The model under review builds one solid part; all positions refer to its coordinate system, in mm. A direction names the side the tool comes from. Round coordinates to 2 decimals unless told otherwise and drop trailing zeros. Write each loop counter-clockwise with the first axis right and the second up, starting at its lowest first coordinate (ties: lowest second). Pieces come first, ordered by that corner, then holes. Notation, with made-up numbers: (54, 14.5) -> (88, 14.5) arc R22 ccw to (88, 43.5) -> close; hole circle Ø8 at (16, -22). An arc over 180 degrees is marked (long way). Return JSON: item names as keys, results as strings. Group by question number.
1. Clearance check with flat-ended pins moving along their axes: P1, Ø1.2, axis at x = 47.5, y = -2, coming from the -Z side; P2, Ø0.8, axis at x = 3.5, z = -111.5, coming from the -Y side; P3, Ø0.8, axis at x = 44.5, z = -88, coming from the -Y side; P4, Ø2, axis at x = 47.5, y = -2, coming from the +Z side. State where each tip first meets the part, or that it passes through.
2. Mouldability with a two-part tool opening along Z and no side actions: class faces 4 (the flat face through (47, -2, -85.5)), 5 (the cylindrical face through (62.67, -1.97, -90.48)), 6 (the flat face through (47, -2, -90.5)), 7 (the flat face through (64, -4, -89)) as pulls with the +Z half, pulls with the -Z half, needs draft (parallel to the pull), parting line crosses it, or undercut.
3. Take a section at A-A, the plane y = -2.5. Give the number of separate pieces and of enclosed holes in the cut face, then the cut area to 3 significant figures.
4. Tool access review of faces 1 (the cylindrical face through (52, -2, -22)), 2 (the flat face through (39, 2, 0)), 3 (the flat face through (47, -2, -24.5)): name each direction out of +Z, -Z, +X, -X, +Y, -Y from which nothing blocks a thin tool from reaching the whole face with its end or side.
5. Take a section at B-B, the plane z = -16. Write out the cut boundary in (x, y), then the cut area to 3 significant figures.
6. Take a section at C-C, the plane x = 27. Write out the cut boundary in (y, z).
7. For line 1 along Z through (x, y) = (49.5, -0.9); line 2 along Z through (x, y) = (3.5, 1.9); line 3 along Z through (x, y) = (51.5, -0.5), list the stretches that pass through material, from the lowest coordinate up. Write a range as from..to.
Autodesk Inventor part; units mm, degrees
ref_plane "YZ Plane" through (0, 0, 0) normal (1, 0, 0) x (0, 1, 0)
ref_plane "XZ Plane" through (0, 0, 0) normal (0, 1, 0) x (-1, 0, 0)
ref_plane "XY Plane" through (0, 0, 0) normal (0, 0, 1) x (1, 0, 0)
sketch "Skizze1" plane through (0, 0, 0) normal (0, 1, 0) x (-1, 0, 0)
  line L0 (0, 0) -> (-80, 0)
  line L1 (-80, 0) -> (-80, -115)
  line L2 (-80, -115) -> (0, -115)
  line L3 (0, -115) -> (0, 0)
  line L4 (-3.5, -3.5) -> (-76.5, -3.5) construction
  line L5 (-76.5, -3.5) -> (-76.5, -111.5) construction
  line L6 (-76.5, -111.5) -> (-3.5, -111.5) construction
  line L7 (-3.5, -111.5) -> (-3.5, -3.5) construction
  circle A0 centre (-3.5, -3.5) radius 0.7
  circle A1 centre (-3.5, -111.5) radius 0.7
  circle A2 centre (-76.5, -111.5) radius 0.7
  circle A3 centre (-76.5, -3.5) radius 0.7
  dimension "d0" = 115
  dimension "d1" = 80
  dimension "d2" = 3.5
  dimension "d3" = 1.4
extrude "Extrusion1" add sketch "Skizze1" along normal blind 4
chamfer "Fasen1" distance 1.2 angle 45 4 edges at (4.2, 4, -3.5) (4.2, 4, -111.5) (77.2, 4, -111.5) (77.2, 4, -3.5)
sketch "Skizze2" plane through (0, 0, 0) normal (0, -1, 0) x (1, 0, 0)
  line L0 (29, -90) -> (46.5, -90) construction
  line L1 (46.5, -90) -> (46.5, -20) construction
  line L2 (46.5, -20) -> (29, -20) construction
  line L3 (29, -20) -> (29, -90) construction
  line L4 (0, -115) -> (0, 0) construction
  line L5 (47.5, -90) -> (65, -90) construction
  line L6 (65, -90) -> (65, -20) construction
  line L7 (65, -20) -> (47.5, -20) construction
  line L8 (47.5, -20) -> (47.5, -90) construction
  line L9 (80, -115) -> (0, -115) construction
  circle A0 centre (31, -88) radius 2.5
  arc A1 (44.5, -85.5) -> (44.5, -90.5) centre (44.5, -88) ccw
  circle A2 centre (63, -88) radius 2.5
  circle A3 centre (31, -22) radius 2.5
  arc A4 (44.5, -19.5) -> (44.5, -24.5) centre (44.5, -22) ccw
  arc A5 (49.5, -24.5) -> (49.5, -19.5) centre (49.5, -22) ccw
  circle A6 centre (63, -22) radius 2.5
  line L10 (31, -88) -> (44.5, -88) construction
  line L11 (44.5, -88) -> (44.5, -22) construction
  line L12 (44.5, -22) -> (31, -22) construction
  line L13 (31, -22) -> (31, -88) construction
  line L14 (49.5, -88) -> (63, -88) construction
  line L15 (63, -88) -> (63, -22) construction
  line L16 (63, -22) -> (49.5, -22) construction
  line L17 (49.5, -22) -> (49.5, -88) construction
  line L18 (44.5, -90.5) -> (49.5, -90.5)
  line L19 (44.5, -85.5) -> (49.5, -85.5)
  line L20 (44.5, -24.5) -> (49.5, -24.5)
  line L21 (44.5, -19.5) -> (49.5, -19.5)
  arc A7 (49.5, -90.5) -> (49.5, -85.5) centre (49.5, -88) ccw
  dimension "d9" = 29
  dimension "d10" = 17.5
  dimension "d11" = 70
  dimension "d12" = 25
  dimension "d13" = 1
  dimension "d14" = 2
  dimension "d15" = 2
  dimension "d16" = 5
extrude "Extrusion2" add sketch "Skizze2" along normal blind 4
sketch "Skizze3" plane through (31, -4, -22) normal (0, -1, 0) x (1, 0, 0)
  circle A0 centre (0, 0) radius 0.7
  arc A1 (13.5, 2.5) -> (13.5, -2.5) centre (13.5, 0) ccw
  circle A2 centre (13.5, 0) radius 0.7
  circle A3 centre (32, 0) radius 2.5
  circle A4 centre (32, 0) radius 0.7
  arc A5 (18.5, -2.5) -> (18.5, 2.5) centre (18.5, 0) ccw
  circle A6 centre (18.5, 0) radius 0.7
  circle A7 centre (0, -66) radius 0.7
  arc A8 (13.5, -63.5) -> (13.5, -68.5) centre (13.5, -66) ccw
  circle A9 centre (13.5, -66) radius 0.7
  arc A10 (18.5, -68.5) -> (18.5, -63.5) centre (18.5, -66) ccw
  circle A11 centre (18.5, -66) radius 0.7
  circle A12 centre (32, -66) radius 0.7
  circle A13 centre (0, 0) radius 2.5
  circle A14 centre (0, -66) radius 2.5
  circle A15 centre (32, -66) radius 2.5
  point P0 (-31, 22)
  dimension "d19" = 1.4
extrude "Extrusion3" cut sketch "Skizze3" against normal blind 5 contours A0 | A2 | A4 | A6 | A7 | A9 | A11 | A12
properties part number "Honigschleuder_Steuerung_Deckel"
Output:
{
 "1": {"P1": "stops at z = -90.5", "P2": "passes through", "P3": "stops at y = 1", "P4": "stops at z = -19.5"},
 "2": {"face 4": "undercut", "face 5": "undercut", "face 6": "pulls with the -Z half", "face 7": "needs draft"},
 "3": {"separate pieces": "6", "enclosed holes": "8", "area": "155 mm^2"},
 "4": {"face 1": "-Y", "face 2": "+Z, +X, -X, +Y, -Y", "face 3": "+X, -X, -Y"},
 "5": {"outline": "(0, 0) -> (80, 0) -> (80, 4) -> (0, 4) -> close", "area": "320 mm^2"},
 "6": {"outline": "(0, -115) -> (4, -115) -> (4, 0) -> (0, 0) -> close"},
 "7": {"line 1": "z = -90.5..-88.7, -87.3..-85.5, -24.5..-22.7, -21.3..-19.5", "line 2": "z = -115..-112.2, -110.8..-4.2, -2.8..0", "line 3": "z = -89.5..-86.5, -23.5..-20.5"}
}
